from build123d import *

# Parameters (mm, degrees)
SKETCH1_W                                       = 215.9
SKETCH1_H                                       = 120.65
BOSS_EXTRUDE1_DEPTH                             = 6.35
CSK_FOR_10_FLAT_HEAD_MACHINE_SCREW1_D           = 5.1054
CSK_FOR_10_FLAT_HEAD_MACHINE_SCREW1_CSINK_D     = 9.779
CSK_FOR_10_FLAT_HEAD_MACHINE_SCREW1_CSINK_ANGLE = 82
CSK_FOR_8_FLAT_HEAD_MACHINE_SCREW1_D            = 4.4958
CSK_FOR_8_FLAT_HEAD_MACHINE_SCREW1_CSINK_D      = 8.4328
CSK_FOR_8_FLAT_HEAD_MACHINE_SCREW1_CSINK_ANGLE  = 82
CSK_FOR_8_FLAT_HEAD_MACHINE_SCREW2_D            = 4.4958
CSK_FOR_8_FLAT_HEAD_MACHINE_SCREW2_CSINK_D      = 8.4328
CSK_FOR_8_FLAT_HEAD_MACHINE_SCREW2_CSINK_ANGLE  = 82
SKETCH10_W                                      = 12.7
SKETCH10_H                                      = 120.65
SKETCH10_H_2                                    = 63.5
CUT_EXTRUDE1_DEPTH                              = 1.524
SKETCH13_W                                      = 24.892
SKETCH13_H                                      = 31.75
CUT_EXTRUDE2_DEPTH                              = 248.405648682
FILLET2_R                                       = 6.35
SKETCH14_W                                      = 12.7
SKETCH14_H                                      = 3.175
CUT_EXTRUDE4_DEPTH                              = 248.405648682
FILLET4_R                                       = 6.35


with BuildPart() as part:
    # Sketch1 → Boss-Extrude1 (new body)
    with BuildSketch(Plane(origin=(0, 0, 0), x_dir=(1, 0, 0), z_dir=(0, 1, 0))):
        with Locations((107.95, 60.325)):
            Rectangle(SKETCH1_W, SKETCH1_H)
    extrude(amount=BOSS_EXTRUDE1_DEPTH)

    # CSK for #10 Flat Head Machine Screw1 (through all)
    with Locations(Plane(origin=(0, 6.35, 0), x_dir=(-1, 0, 0), z_dir=(0, 1, 0))):
        with Locations((-6.35, -111.125), (-209.55, -111.125), (-209.55, -9.525), (-6.35, -9.525), (-6.35, -60.325), (-209.55, -60.325), (-158.75, -111.125), (-57.15, -111.125), (-57.15, -9.525), (-158.75, -9.525)):
            CounterSinkHole(CSK_FOR_10_FLAT_HEAD_MACHINE_SCREW1_D / 2, CSK_FOR_10_FLAT_HEAD_MACHINE_SCREW1_CSINK_D / 2, counter_sink_angle=CSK_FOR_10_FLAT_HEAD_MACHINE_SCREW1_CSINK_ANGLE)

    # CSK for #8 Flat Head Machine Screw1 (through all)
    with Locations(Plane.XZ):
        with Locations((37.592, -12.7), (37.592, -60.325), (37.592, -107.95)):
            csk_for_8_flat_head_machine_screw1 = CounterSinkHole(CSK_FOR_8_FLAT_HEAD_MACHINE_SCREW1_D / 2, CSK_FOR_8_FLAT_HEAD_MACHINE_SCREW1_CSINK_D / 2, counter_sink_angle=CSK_FOR_8_FLAT_HEAD_MACHINE_SCREW1_CSINK_ANGLE)

    # Mirror1: CSK for #8 Flat Head Machine Screw1 across plane
    add(csk_for_8_flat_head_machine_screw1.mirror(Plane.ZY.offset(-107.95)), mode=Mode.SUBTRACT)

    # CSK for #8 Flat Head Machine Screw2 (through all)
    with Locations(Plane.XZ):
        with Locations((147.335875, -8.636), (147.335875, -40.386)):
            CounterSinkHole(CSK_FOR_8_FLAT_HEAD_MACHINE_SCREW2_D / 2, CSK_FOR_8_FLAT_HEAD_MACHINE_SCREW2_CSINK_D / 2, counter_sink_angle=CSK_FOR_8_FLAT_HEAD_MACHINE_SCREW2_CSINK_ANGLE)

    # Sketch10 → Cut-Extrude1 (cut)
    with BuildSketch(Plane(origin=(0, 6.35, 0), x_dir=(1, 0, 0), z_dir=(0, 1, 0))):
        with Locations((37.592, 60.325)):
            Rectangle(SKETCH10_W, SKETCH10_H)
        with Locations((178.308, 60.325)):
            Rectangle(SKETCH10_W, SKETCH10_H)
        with Locations((147.335875, 31.75)):
            Rectangle(SKETCH10_W, SKETCH10_H_2)
    extrude(amount=-CUT_EXTRUDE1_DEPTH, mode=Mode.SUBTRACT)

    # Sketch13 → Cut-Extrude2 (cut, through all)
    with BuildSketch(Plane(origin=(0, 6.35, 0), x_dir=(1, 0, 0), z_dir=(0, 1, 0))):
        with Locations((12.446, 85.725)):
            Rectangle(SKETCH13_W, SKETCH13_H)
        with Locations((12.446, 34.925)):
            Rectangle(SKETCH13_W, SKETCH13_H)
    cut_extrude2 = extrude(amount=-CUT_EXTRUDE2_DEPTH, mode=Mode.SUBTRACT)

    # Mirror4: Cut-Extrude2 across plane
    add(cut_extrude2.mirror(Plane.ZY.offset(-107.95)), mode=Mode.SUBTRACT)

    # Fillet2
    fillet2_edges = [part.edges().sort_by_distance(p)[0] for p in [
        (0, 3.175, -69.85),
        (0, 3.175, -101.6),
        (24.892, 3.175, -101.6),
        (24.892, 3.175, -69.85),
        (0, 3.175, -19.05),
        (0, 3.175, -50.8),
        (24.892, 3.175, -50.8),
        (24.892, 3.175, -19.05),
        (215.9, 3.175, -101.6),
        (215.9, 3.175, -69.85),
        (191.008, 3.175, -69.85),
        (191.008, 3.175, -101.6),
        (215.9, 3.175, -50.8),
        (215.9, 3.175, -19.05),
        (191.008, 3.175, -19.05),
        (191.008, 3.175, -50.8),
        (0, 3.175, -120.65),
        (215.9, 3.175, -120.65),
        (215.9, 3.175, 0),
        (0, 3.175, 0),
    ]]
    fillet(fillet2_edges, radius=FILLET2_R)

    # Sketch14 → Cut-Extrude4 (cut, through all)
    with BuildSketch(Plane(origin=(0, 6.35, 0), x_dir=(1, 0, 0), z_dir=(0, 1, 0))):
        Polygon((146.558, 114.3), (69.342, 114.3), (69.342, 101.6), (50.292, 101.6), (50.292, 19.05), (69.342, 19.05), (69.342, 6.35), (134.635875, 6.35), (134.635875, 19.05), (134.635875, 60.325), (140.985875, 60.325), (140.985875, 63.5), (153.685875, 63.5), (153.685875, 60.325), (165.608, 60.325), (165.608, 101.6), (146.558, 101.6), align=None)
        with Locations((147.335875, 61.9125)):
            Rectangle(SKETCH14_W, SKETCH14_H)
    extrude(amount=-CUT_EXTRUDE4_DEPTH, mode=Mode.SUBTRACT)

    # Fillet4
    fillet4_edges = [part.edges().sort_by_distance(p)[0] for p in [
        (165.608, 3.175, -101.6),
        (134.635875, 3.175, -6.35),
        (69.342, 3.175, -6.35),
        (50.292, 3.175, -19.05),
        (50.292, 3.175, -101.6),
        (69.342, 3.175, -114.3),
        (146.558, 3.175, -114.3),
        (69.342, 3.175, -19.05),
        (69.342, 3.175, -101.6),
        (146.558, 3.175, -101.6),
        (165.608, 3.175, -60.325),
        (134.635875, 3.175, -60.325),
    ]]
    fillet(fillet4_edges, radius=FILLET4_R - 0.0001)  # a hair under: the kernel refuses the full size


solid = part.part
Check sheet for the modelled part. Datum: model origin and axes. Units: mm. A direction names the side the tool comes from. Round coordinates to 2 decimals unless told otherwise and drop trailing zeros. Loops run counter-clockwise (first coordinate to the right, second up) from the corner with the lowest first, then second, coordinate; pieces in that order, holes last.
1. Scan lines: probe 1 along X at (y, z) = (4.3, -12.7); probe 2 along X at (y, z) = (5.25, -83); probe 3 along Z at (x, y) = (16.5, 1.5). Record each from-to range of solid material in increasing order.
2. Sectioned sample at B-B on y = 1. Give the number of separate pieces and of enclosed holes in the cut face, and give its area (3 significant figures).
3. Gauge pin test, flat ends, axial feed: pin 1 Ø4.5 at (x, z) = (57.15, -9.525) entering from +Y; pin 2 Ø1.9 at (y, z) = (3, -39) entering from +X. Record the tip position at first contact, or that the pin passes through.
4. Set-up check for faces 1 (the flat face through (40, 4.826, -61)), 2 (the cylindrical face through (192.82, 3.13, -71.76)), 3 (the flat face through (102, 3, -6.35)): record each of +Z, -Z, +X, -X, +Y, -Y from which the full face is reachable in a straight line by a thin tool's end or side.
5. Sectioned sample at A-A on z = -73.5. Record the boundary of the cut face in (x, y), and give its area (3 significant figures).
6. Mould release check, pull along Z, two halves, no side actions. Record for faces 4 (the flat face through (107, 3, -120.65)), 5 (the cylindrical face through (213.99, 3.22, -1.81)), 6 (the flat face through (0, 3, -9)), 7 (the flat face through (12, 3, -101.6)): released by +Z, released by -Z, zero draft, split by the parting line, or undercut.
Recorded:
1. probe 1: x = 0 to 35.34, 39.84 to 69.34, 134.64 to 176.06, 180.56 to 215.9
1. probe 2: x = 24.89 to 31.24, 43.94 to 50.29, 165.61 to 171.96, 184.66 to 191.01
1. probe 3: z = -120.65 to -101.6, -69.85 to -50.8, -19.05 to 0
2. separate pieces: 1
2. enclosed holes: 19
2. area: 12,300 mm2
3. pin 1: passes through
3. pin 2: stops at x = 191.01
4. face 1: +Z, -Z, +Y
4. face 2: +X, +Y, -Y
4. face 3: +Y, -Y
5. outline: (24.29, 0) - (50.29, 0) - (50.29, 6.35) - (43.94, 6.35) - (43.94, 4.83) - (31.24, 4.83) - (31.24, 6.35) - (24.29, 6.35) - close; (165.61, 0) - (191.61, 0) - (191.61, 6.35) - (184.66, 6.35) - (184.66, 4.83) - (171.96, 4.83) - (171.96, 6.35) - (165.61, 6.35) - close
5. area: 292 mm2
6. face 4: released by -Z
6. face 5: released by +Z
6. face 6: zero draft
6. face 7: undercut
